Design review of the part built by this model. Coordinates are the model's own, in mm. A direction names the side the tool comes from. Coordinates: 2 decimals unless noted, no trailing zeros. Order: outer loops, then holes, each group sorted by start corner. A loop starts at its lowest first (then second) coordinate and runs counter-clockwise, first axis right, second up. Notation, with made-up numbers: (20, 51) - (36, 51) arc R17 ccw to (36, 76) - close; hole circle Ø1 at (78, 6.5). An arc over 180 degrees is marked (long way). Write each question's results on one line, items separated by ' | '. Start each with the question number.
```python
from build123d import *

# Parameters (mm, degrees)
SKETCH012_W     = 17
SKETCH012_H     = 21
PAD009_DEPTH    = 30
SKETCH013_W     = 13.1
SKETCH013_H     = 17
POCKET001_DEPTH = 26.7
SKETCH014_W     = 11.5
SKETCH014_H     = 1.2
SKETCH014_W_2   = 3.205285
SKETCH014_H_2   = 1.736194
POCKET002_DEPTH = 27.8
SKETCH016_R     = 0.6
POCKET003_DEPTH = 27
SKETCH022_W     = 0.6
SKETCH022_H     = 3
POCKET005_DEPTH = 3


with BuildPart() as part:
    # Sketch012 → Pad009 (new body)
    with BuildSketch(Plane.XZ):
        with Locations((1.5, 2)):
            Rectangle(SKETCH012_W, SKETCH012_H)
    extrude(amount=PAD009_DEPTH)

    # Sketch013 (on Face5 of Pad009) → Pocket001 (cut)
    with BuildSketch(Plane(origin=(0, 0, 0), x_dir=(1, 0, 0), z_dir=(0, 1, 0))):
        with Locations((2.05, -2)):
            Rectangle(SKETCH013_W, SKETCH013_H)
    extrude(amount=-POCKET001_DEPTH, mode=Mode.SUBTRACT)

    # Sketch014 (on Face4 of Pocket001) → Pocket002 (cut)
    with BuildSketch(Plane(origin=(0, 0, 0), x_dir=(1, 0, 0), z_dir=(0, 1, 0))):
        Rectangle(SKETCH014_W, SKETCH014_H)
        with Locations((9.189982, -4.640042)):
            Rectangle(SKETCH014_W_2, SKETCH014_H_2)
    extrude(amount=-POCKET002_DEPTH, mode=Mode.SUBTRACT)

    # Sketch016 (on Face6 of Pocket002) → Pocket003 (cut)
    with BuildSketch(Plane(origin=(0, 0, -8.5), x_dir=(1, 0, 0), z_dir=(0, 0, -1))):
        with Locations((0, 3)):
            Circle(SKETCH016_R)
    extrude(amount=-POCKET003_DEPTH, mode=Mode.SUBTRACT)

    # Sketch022 (on Face21 of Pocket003) → Pocket005 (cut)
    with BuildSketch(Plane(origin=(0, -26.7, 0), x_dir=(1, 0, 0), z_dir=(0, 1, 0))):
        with Locations((0, -9)):
            Rectangle(SKETCH022_W, SKETCH022_H)
    extrude(amount=-POCKET005_DEPTH, mode=Mode.SUBTRACT)


solid = part.part
```
(1) Take a section at C-C (x = 1.25). State the section outline as (y, z) points, plus the area to 3 significant figures.
(2) Take a section at B-B (z = 1.5). State the section outline as (x, y) points, plus the area to 3 significant figures.
(3) To check wall thickness, follow line 1 along Z through (x, y) = (8.5, -10); line 2 along X through (y, z) = (-22.75, -2); line 3 along X through (y, z) = (-3, -7.5). State the ranges of each line that lie inside material, in increasing order. Write a range as [from, to].
(4) Take a section at A-A (y = -3). State the section outline as (x, z) points, plus the area to 3 significant figures.
(5) Tool access review of faces 4 (the face through (2, -13, -6.5)), 5 (the face through (7.587, -27, 5)), 6 (the face through (1, -15, 12.5)): name each direction out of +Z, -Z, +X, -X, +Y, -Y from which nothing blocks a thin tool from reaching the whole face with its end or side.
(6) Take a section at D-D (y = -25.5). State the section outline as (x, z) points, plus the area to 3 significant figures.
(7) Mouldability with a two-part tool opening along X and no side actions: class faces 1 (the face through (-7, -15, 2)), 2 (the face through (10, -15, 2)), 3 (the face through (-4.5, -13, 6)) as +X half, -X half, draft (parallel to the pull), parting line (faces both ways), or undercut.
(8) Clearance check with flat-ended pins moving along their axes: pin 1 (1 mm diameter, centred on x = -0.5, z = 0, fed in from +Y); pin 2 (3 mm diameter, centred on x = 0, z = 3, fed in from +Y). State where each tip first meets the part, or that it passes through.
Worked out:
1) outline: (-30, -8.5) - (0, -8.5) - (0, -6.5) - (-26.7, -6.5) - (-26.7, -0.6) - (-27.8, -0.6) - (-27.8, 0.6) - (-26.7, 0.6) - (-26.7, 10.5) - (0, 10.5) - (0, 12.5) - (-30, 12.5) - close | area: 175 mm^2
2) outline: (-7, -30) - (10, -30) - (10, 0) - (8.6, 0) - (8.6, -26.7) - (-4.5, -26.7) - (-4.5, 0) - (-7, 0) - close | area: 160 mm^2
3) line 1: [-8.5, -6.5], [10.5, 12.5] | line 2: [-7, -4.5], [8.6, 10] | line 3: [-7, -0.6], [0.6, 10]
4) outline: (-7, -8.5) - (-0.6, -8.5) - (-0.6, -6.5) - (-4.5, -6.5) - (-4.5, -0.6) - (-5.75, -0.6) - (-5.75, 0.6) - (-4.5, 0.6) - (-4.5, 10.5) - (-0.6, 10.5) - (-0.6, 12.5) - (-7, 12.5) - close; (0.6, -8.5) - (10, -8.5) - (10, 3.77) - (8.6, 3.77) - (8.6, -6.5) - (0.6, -6.5) - close; (0.6, 10.5) - (8.6, 10.5) - (8.6, 5.51) - (10, 5.51) - (10, 12.5) - (0.6, 12.5) - close | area: 126 mm^2
5) face 4: +Y | face 5: +X, +Y | face 6: +Z, +X, -X, +Y, -Y
6) outline: (-7, -8.5) - (10, -8.5) - (10, 3.77) - (8.6, 3.77) - (8.6, -6.5) - (-4.5, -6.5) - (-4.5, -0.6) - (-5.75, -0.6) - (-5.75, 0.6) - (-4.5, 0.6) - (-4.5, 10.5) - (8.6, 10.5) - (8.6, 5.51) - (10, 5.51) - (10, 12.5) - (-7, 12.5) - close | area: 130 mm^2
7) face 1: -X half | face 2: +X half | face 3: undercut
8) pin 1: y = -27.8 | pin 2: y = -26.7
